Check sheet for the drawn part. Datum: minimum x, y, z corner. Units: mm. A direction names the side the tool comes from. Give positions to 0.01 mm unless a question says otherwise; leave off trailing zeros. Order: outer loops, then holes, each group sorted by start corner. A loop starts at its lowest first (then second) coordinate and runs counter-clockwise, first axis right, second up. Notation, with made-up numbers: (34, -4) -> (69, -4) arc R25 cw to (69, 34) -> close; hole circle Ø2 at (20, 87.25). An arc over 180 degrees is marked (long way). Answer in a Markdown table with one row per item. Add a question column.
(1) Go/stop test with flat-tipped pins: pin 1 (1.5 mm diameter, centred on x = 15.5, y = 11, fed in from +Z); pin 2 (10 mm diameter, centred on x = 6.5, z = 15, fed in from +Y); pin 3 (3 mm diameter, centred on x = 7.5, y = 17.5, fed in from +Z); pin 4 (1 mm diameter, centred on x = 17.5, z = 4, fed in from +Y). Record where each tip stops, or that it passes through.
(2) Cross-section at A-A (z = 17.5). Record the cut outline in (x, y), then the cut area to 3 significant figures.
(3) Cross-section at B-B (x = 17.5). Record the cut outline in (y, z), then the cut area to 3 significant figures.
(4) Cross-section at D-D (y = 6.5). Record the cut outline in (x, z).
(5) Release check for a two-part mould opening along Y. For the marked faces 3, 4 and 5 record: released by +Y, released by -Y, zero draft, split by the parting line, or undercut.
(6) Thickness scan on L1, parallel to Y at x = 7.5, z = 1.9; L2, parallel to X at y = 17.25, z = 4.25; L3, parallel to Y at x = 23, z = 19.75. Record the ranges inside material, lowest first. Write a range as [from, to].
(7) Set-up check for the marked faces 1 and 2: record each of +Z, -Z, +X, -X, +Y, -Y from which the full face is reachable in a straight line by a thin tool's end or side.
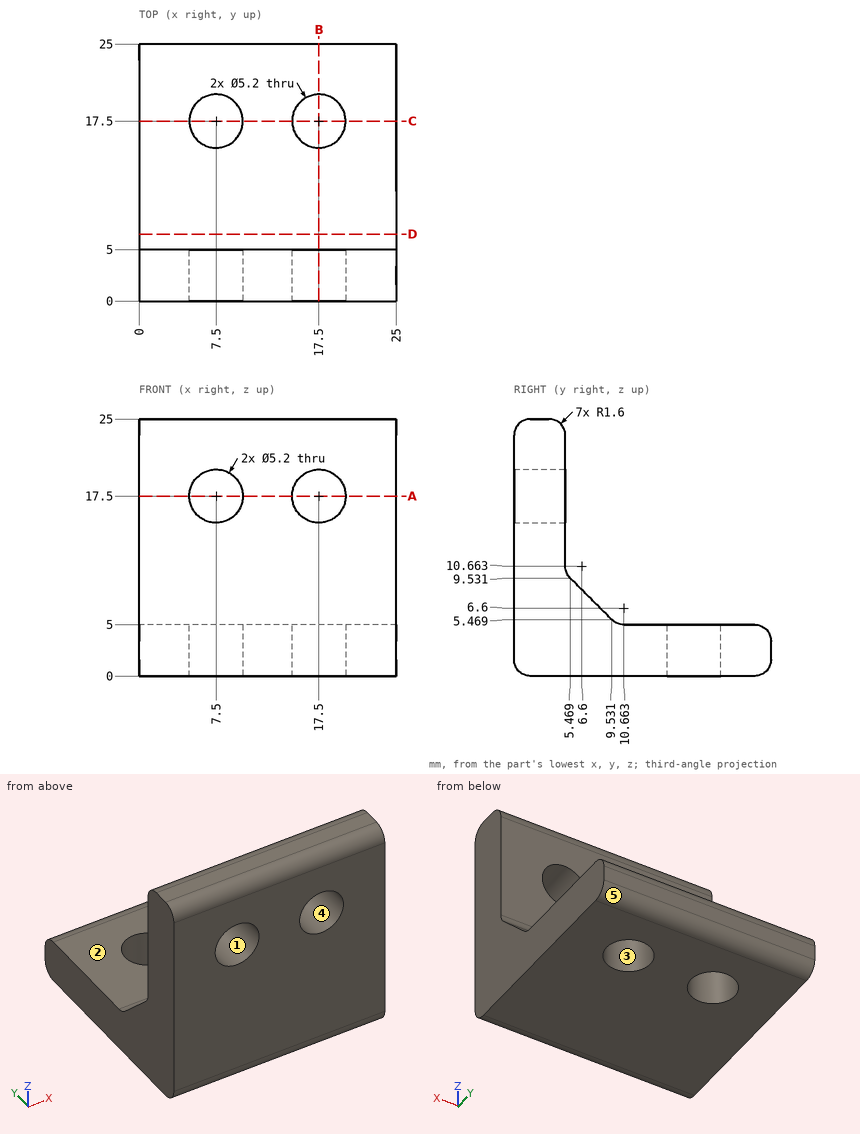
Answer below:
| question | item | result |
|---|---|---|
| 1 | pin 1 | stops at z = 5.05 |
| 1 | pin 2 | stops at y = 5.14 |
| 1 | pin 3 | passes through |
| 1 | pin 4 | stops at y = 25 |
| 2 | outline | (0, 0) -> (4.9, 0) -> (4.9, 5) -> (0, 5) -> close; (10.1, 0) -> (14.9, 0) -> (14.9, 5) -> (10.1, 5) -> close; (20.1, 0) -> (25, 0) -> (25, 5) -> (20.1, 5) -> close |
| 2 | area | 73.0 mm² |
| 3 | outline | (0, 1.6) arc R1.6 ccw to (1.6, 0) -> (14.9, 0) -> (14.9, 5) -> (10.66, 5) arc R1.6 cw to (9.53, 5.47) -> (5.47, 9.53) arc R1.6 cw to (5, 10.66) -> (5, 14.9) -> (0, 14.9) -> close; (0, 20.1) -> (5, 20.1) -> (5, 23.4) arc R1.6 ccw to (3.4, 25) -> (1.6, 25) arc R1.6 ccw to (0, 23.4) -> close; (20.1, 0) -> (23.4, 0) arc R1.6 ccw to (25, 1.6) -> (25, 3.4) arc R1.6 ccw to (23.4, 5) -> (20.1, 5) -> close |
| 3 | area | 183 mm² |
| 4 | outline | (0, 0) -> (25, 0) -> (25, 8.5) -> (0, 8.5) -> close |
| 5 | face 3 | undercut |
| 5 | face 4 | zero draft |
| 5 | face 5 | released by +Y |
| 6 | L1 | y = [0, 14.9], [20.1, 25] |
| 6 | L2 | x = [0, 4.91], [10.09, 14.91], [20.09, 25] |
| 6 | L3 | y = [0, 5] |
| 7 | face 1 | +Y, -Y |
| 7 | face 2 | +Z, +X, -X, +Y |
